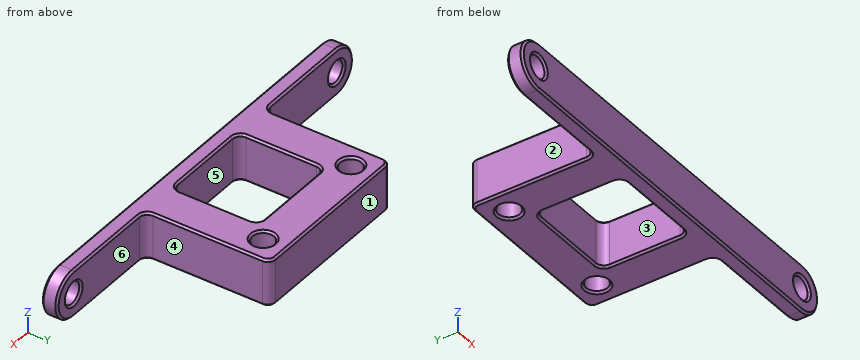
```python
from build123d import *

# Parameters (mm, degrees)
SKETCH2_R               = 2.1828125
BOSS_EXTRUDE1_DEPTH     = 3.175
SKETCH3_W               = 36.843225838
SKETCH3_H               = 9.525
BOSS_EXTRUDE2_DEPTH     = 25.4
CUT_EXTRUDE1_DEPTH      = 53.3875
CUT_EXTRUDE1_DEPTH_BACK = 53.3875
SKETCH4_R               = 2.1828125
SKETCH4_W               = 0.959112919
SKETCH4_H               = 25.4
SKETCH4_W_2             = 19.05
SKETCH4_H_2             = 17.4625
FILLET1_R               = 1.5875
CHAMFER1_SIZE           = 0.396875


with BuildPart() as part:
    # Sketch2 → Boss-Extrude1 (new body)
    with BuildSketch(Plane(origin=(0, 0, 0), x_dir=(1, 0, 0), z_dir=(0, 1, 0))):
        with BuildLine():
            Line((-38.1, 4.7625), (38.1, 4.7625))
            ThreePointArc((38.1, 4.7625), (42.8625, 0), (38.1, -4.7625))
            Line((38.1, -4.7625), (-38.1, -4.7625))
            ThreePointArc((-38.1, -4.7625), (-42.8625, 0), (-38.1, 4.7625))
        make_face()
        with Locations(Location((-38.1, 0, 0), (0, 0, 270))):
            Circle(SKETCH2_R, mode=Mode.SUBTRACT)
        with Locations(Location((38.1, 0, 0), (0, 0, 270))):
            Circle(SKETCH2_R, mode=Mode.SUBTRACT)
    extrude(amount=BOSS_EXTRUDE1_DEPTH)

    # Sketch3 → Boss-Extrude2 (add)
    with BuildSketch(Plane(origin=(0, 3.175, 0), x_dir=(1, 0, 0), z_dir=(0, 1, 0))):
        Rectangle(SKETCH3_W, SKETCH3_H)
    extrude(amount=BOSS_EXTRUDE2_DEPTH)

    # Sketch4 → Cut-Extrude1 (cut, two sides: drawn at the far end of the back side and taken through both)
    with BuildSketch(Plane.XY.offset(4.7625).offset(-CUT_EXTRUDE1_DEPTH_BACK)):
        with Locations((-12.7, 23.8125)):
            Circle(SKETCH4_R)
        with Locations((12.7, 23.8125)):
            Circle(SKETCH4_R)
        with Locations((-17.94205646, 15.875)):
            Rectangle(SKETCH4_W, SKETCH4_H)
        with Locations((17.94205646, 15.875)):
            Rectangle(SKETCH4_W, SKETCH4_H)
        with Locations((0, 11.90625)):
            Rectangle(SKETCH4_W_2, SKETCH4_H_2)
    extrude(amount=CUT_EXTRUDE1_DEPTH + CUT_EXTRUDE1_DEPTH_BACK, mode=Mode.SUBTRACT)

    # Fillet1
    fillet1_edges = [part.edges().sort_by_distance(p)[0] for p in [
        (-17.4625, 3.175, 0),
        (-17.4625, 28.575, 0),
        (17.4625, 28.575, 0),
        (17.4625, 3.175, 0),
        (-9.525, 3.175, 0),
        (-9.525, 20.6375, 0),
        (9.525, 20.6375, 0),
        (9.525, 3.175, 0),
    ]]
    fillet(fillet1_edges, radius=FILLET1_R)

    # Chamfer1
    chamfer1_edges = [part.edges().sort_by_distance(p)[0] for p in [
        (0, 28.575, -4.7625),
        (0, 28.575, 4.7625),
        (0, 3.175, 4.7625),
        (-9.525, 11.90625, 4.7625),
        (0, 20.6375, 4.7625),
        (9.525, 11.90625, 4.7625),
        (-17.4625, 15.875, 4.7625),
        (28.575, 3.175, 4.7625),
        (17.4625, 15.875, 4.7625),
        (16.997532015, 28.110032015, 4.7625),
        (-16.997532015, 28.110032015, 4.7625),
        (-17.4625, 15.875, -4.7625),
        (0, 20.6375, -4.7625),
        (-9.525, 11.90625, -4.7625),
        (0, 3.175, -4.7625),
        (9.525, 11.90625, -4.7625),
        (-28.575, 3.175, -4.7625),
        (17.4625, 15.875, -4.7625),
        (16.997532015, 28.110032015, -4.7625),
        (-16.997532015, 28.110032015, -4.7625),
        (-38.1, 0, -2.1828125),
        (-17.927467985, 3.639967985, 4.7625),
        (-38.1, 3.175, -2.1828125),
        (-17.927467985, 3.639967985, -4.7625),
        (17.927467985, 3.639967985, 4.7625),
        (17.927467985, 3.639967985, -4.7625),
        (-9.060032015, 20.172532015, 4.7625),
        (42.8625, 3.175, 0),
        (-9.060032015, 20.172532015, -4.7625),
        (9.060032015, 20.172532015, 4.7625),
        (9.060032015, 20.172532015, -4.7625),
        (9.060032015, 3.639967985, 4.7625),
        (9.060032015, 3.639967985, -4.7625),
        (-9.060032015, 3.639967985, 4.7625),
        (-9.060032015, 3.639967985, -4.7625),
        (38.1, 0, -2.1828125),
        (38.1, 3.175, -2.1828125),
        (28.575, 3.175, -4.7625),
        (10.5171875, 23.8125, -4.7625),
        (10.5171875, 23.8125, 4.7625),
        (-42.8625, 3.175, 0),
        (0, 0, -4.7625),
        (42.8625, 0, 0),
        (0, 0, 4.7625),
        (-42.8625, 0, 0),
        (-14.8828125, 23.8125, -4.7625),
        (-14.8828125, 23.8125, 4.7625),
        (-28.575, 3.175, 4.7625),
    ]]
    chamfer(chamfer1_edges, length=CHAMFER1_SIZE)


solid = part.part
```
Check sheet for the modelled part. Datum: model origin and axes. Units: mm. Face numbers are marked on the shaded views. A direction names the side the tool comes from. Give positions to 0.01 mm unless a question says otherwise; leave off trailing zeros. Order: outer loops, then holes, each group sorted by start corner. A loop starts at its lowest first (then second) coordinate and runs counter-clockwise, first axis right, second up. Notation, with made-up numbers: M 36,-6.75 L 41,-6.75 A28 ccw 41,32.25 Z; hole C 38.25,51.5 d9. An arc over 180 degrees is marked long. Answer in a Markdown table with one row per item.
1) Cross-section at C-C, the plane x = 22. Enter the section's corners in (y, z) (1 decimal).
Filled sheet:
| item | result |
|---|---|
| outline | M 0,-4.4 L 0.4,-4.8 L 2.8,-4.8 L 3.2,-4.4 L 3.2,4.4 L 2.8,4.8 L 0.4,4.8 L 0,4.4 Z |
2) Release check for a two-part mould opening along X. For the marked faces 4, 5 and 6 record: +X half, -X half, draft (parallel to the pull), parting line (faces both ways), or undercut.
Filled sheet:
| item | result |
|---|---|
| face 4 | +X half |
| face 5 | undercut |
| face 6 | draft |
3) Cross-section at B-B, the plane y = 9.25. Enter the section's corners in (x, z) (1 decimal), plus the area to 3 significant figures.
Filled sheet:
| item | result |
|---|---|
| outline | M -17.5,-4.4 L -17.1,-4.8 L -9.9,-4.8 L -9.5,-4.4 L -9.5,4.4 L -9.9,4.8 L -17.1,4.8 L -17.5,4.4 Z; M 9.5,-4.4 L 9.9,-4.8 L 17.1,-4.8 L 17.5,-4.4 L 17.5,4.4 L 17.1,4.8 L 9.9,4.8 L 9.5,4.4 Z |
| area | 151 mm2 |
4) Access from +Z, -Z, +X, -X, +Y, -Y to the whole of each face (thin tool, end or side, straight path). Record for the marked faces 1, 2 and 3.
Filled sheet:
| item | result |
|---|---|
| face 1 | +Z, -Z, +X, -X, +Y |
| face 2 | +Z, -Z, -X, +Y |
| face 3 | +Z, -Z |
5) Gauge pin test, flat ends, axial feed: P1, Ø4.5, axis at y = 15, z = -2, coming from the +X side; P2, Ø2, axis at y = 14.5, z = -0.5, coming from the -X side; P3, Ø3.5, axis at x = 12.7, y = 23.81, coming from the -Z side; P4, Ø5.5, axis at x = 38.1, z = 0, coming from the +Y side (3 decimals). Record the tip position at first contact, or that the pin passes through.
Filled sheet:
| item | result |
|---|---|
| P1 | stops at x = 17.46 |
| P2 | stops at x = -17.46 |
| P3 | passes through |
| P4 | stops at y = 3.175 |
6) Cross-section at D-D, the plane z = 0. Count the separate pieces of the cut face and the enclosed holes in it, plus the area to 3 significant figures.
Filled sheet:
| item | result |
|---|---|
| separate pieces | 3 |
| enclosed holes | 3 |
| area | 770 mm2 |
7) Cross-section at A-A, the plane x = 12.7. Enter the section's corners in (y, z) (1 decimal).
Filled sheet:
| item | result |
|---|---|
| outline | M 0,-4.4 L 0.4,-4.8 L 21.2,-4.8 L 21.6,-4.4 L 21.6,4.4 L 21.2,4.8 L 0.4,4.8 L 0,4.4 Z; M 26,-4.4 L 26.4,-4.8 L 28.2,-4.8 L 28.6,-4.4 L 28.6,4.4 L 28.2,4.8 L 26.4,4.8 L 26,4.4 Z |
8) Thickness scan on L1, parallel to X at y = 1.4, z = 0; L2, parallel to X at y = 23.75, z = 4; L3, parallel to Y at x = 3, z = 4 (1 decimal). Record the ranges inside material, lowest first. Write a range as [from, to].
Filled sheet:
| item | result |
|---|---|
| L1 | x = [-42.86, -40.28], [-35.92, 35.92], [40.28, 42.86] |
| L2 | x = [-17.46, -14.88], [-10.52, 10.52], [14.88, 17.46] |
| L3 | y = [0, 3.2], [20.6, 28.6] |
